Check sheet for the drawn part. Datum: minimum x, y, z corner. Units: mm. A direction names the side the tool comes from. Give positions to 0.01 mm unless a question says otherwise; leave off trailing zeros. Loops run counter-clockwise (first coordinate to the right, second up) from the corner with the lowest first, then second, coordinate; pieces in that order, holes last.
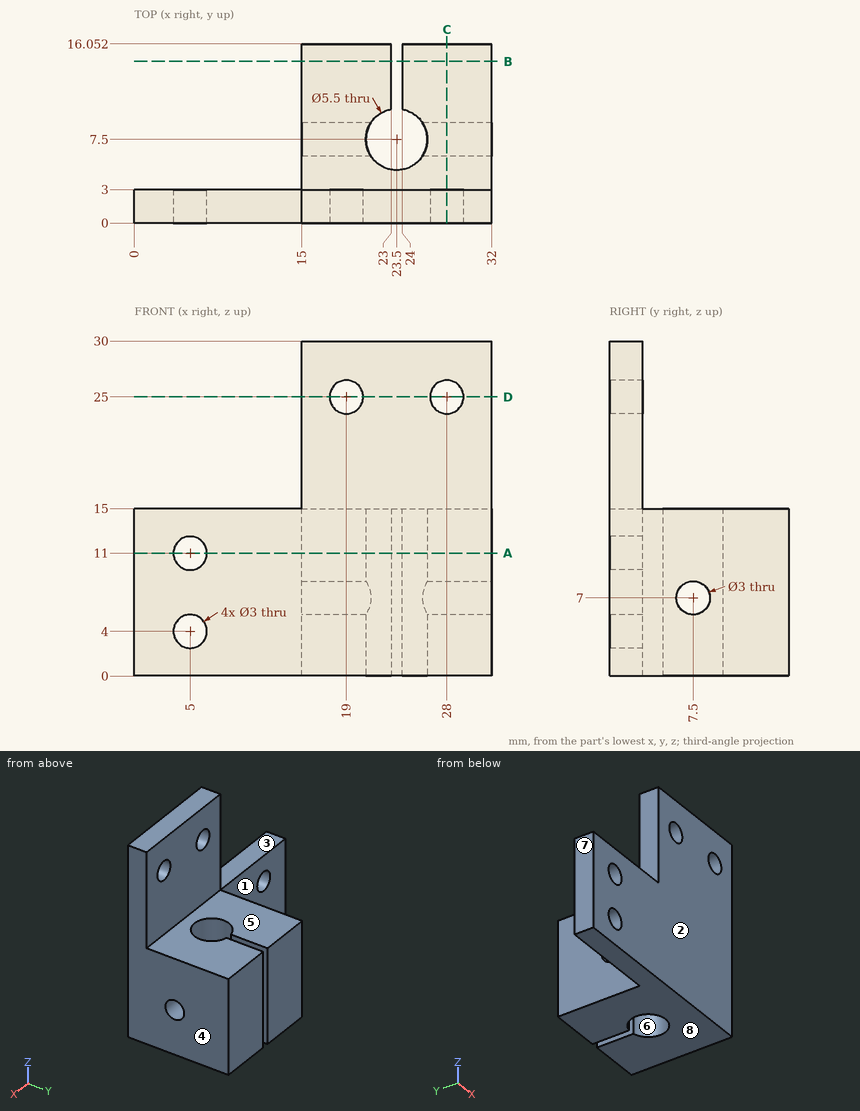
(1) Section check B-B on y = 14.5. Record the boundary of the cut face in (x, z).
(2) Section check C-C on x = 28. Record the boundary of the cut face in (y, z).
(3) Gauge pin test, flat ends, axial feed: pin 1 Ø4 at (x, y) = (24.5, 8.5) entering from +Z; pin 2 Ø3.5 at (y, z) = (7.5, 7) entering from +X; pin 3 Ø12 at (x, z) = (8.5, 10) entering from +Y; pin 4 Ø3.5 at (y, z) = (2, 26) entering from -X. Record the tip position at first contact, or that the pin passes through.
(4) Material ranges on line 1 (Z direction, x = 5, y = 1.35); line 2 (Z direction, x = 28, y = 2.4); line 3 (X direction, y = 15, z = 13), recorded low to high.
(5) Access from +Z, -Z, +X, -X, +Y, -Y to the whole of each face (thin tool, end or side, straight path). Record for the marked faces 1, 2, 3, 4 and 5.
(6) Section check A-A on z = 11. Record the boundary of the cut face in (x, y), plus the area to 3 significant figures.
(7) Release check for a two-part mould opening along X. For the marked faces 6, 7 and 8 record: pulls with the +X half, pulls with the -X half, needs draft (parallel to the pull), parting line crosses it, or undercut.
(8) Section check D-D on z = 25. Record the boundary of the cut face in (x, y), plus the area to 3 significant figures.
Computed values:
1. outline: (15, 0) - (23, 0) - (23, 15) - (15, 15) - close; (24, 0) - (32, 0) - (32, 15) - (24, 15) - close
2. outline: (0, 0) - (16.05, 0) - (16.05, 15) - (3, 15) - (3, 23.5) - (0, 23.5) - close; (0, 26.5) - (3, 26.5) - (3, 30) - (0, 30) - close; hole circle Ø3 at (7.5, 7)
3. pin 1: stops at z = 15
3. pin 2: stops at x = 32
3. pin 3: stops at y = 3
3. pin 4: stops at x = 15
4. line 1: z = 0 to 2.5, 5.5 to 9.5, 12.5 to 15
4. line 2: z = 0 to 23.5, 26.5 to 30
4. line 3: x = 15 to 23, 24 to 32
5. face 1: +Z, -Z, -X, +Y
5. face 2: +Z, -Z, +X, -X, -Y
5. face 3: +Z, -X, +Y, -Y
5. face 4: +Z, -Z, +X, +Y, -Y
5. face 5: +Z, +X, -X, +Y
6. outline: (0, 0) - (3.5, 0) - (3.5, 3) - (0, 3) - close; (6.5, 0) - (32, 0) - (32, 16.05) - (24, 16.05) - (24, 10.2) arc R2.75 cw (long way) to (23, 10.2) - (23, 16.05) - (15, 16.05) - (15, 3) - (6.5, 3) - close
6. area: 279 mm2
7. face 6: undercut
7. face 7: pulls with the -X half
7. face 8: needs draft
8. outline: (15, 0) - (17.5, 0) - (17.5, 3) - (15, 3) - close; (20.5, 0) - (26.5, 0) - (26.5, 3) - (20.5, 3) - close; (29.5, 0) - (32, 0) - (32, 3) - (29.5, 3) - close
8. area: 33.0 mm2
